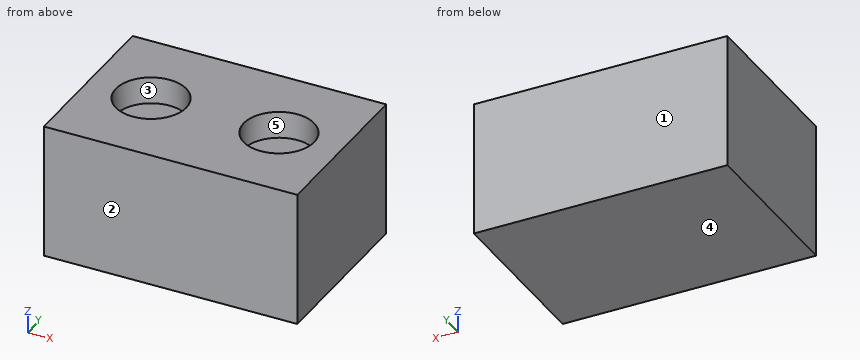
```python
from build123d import *

# Parameters (mm, degrees)
CROQUIS1_W              = 18.8
CROQUIS1_H              = 12.8
SALIENTE_EXTRUIR1_DEPTH = 10
CROQUIS2_R              = 2.614642897
CORTAR_EXTRUIR1_DEPTH   = 2


with BuildPart() as part:
    # Croquis1 → Saliente-Extruir1 (new body)
    with BuildSketch(Plane.XY):
        Rectangle(CROQUIS1_W, CROQUIS1_H)
    extrude(amount=SALIENTE_EXTRUIR1_DEPTH)

    # Croquis2 → Cortar-Extruir1 (cut)
    with BuildSketch(Plane.XY.offset(10)):
        with Locations((-4.740668899, 0)):
            Circle(CROQUIS2_R)
    cortar_extruir1 = extrude(amount=-CORTAR_EXTRUIR1_DEPTH, mode=Mode.SUBTRACT)

    # Simetría1: Cortar-Extruir1 across plane
    add(cortar_extruir1.mirror(Plane(origin=(0, 0, 0), x_dir=(0, 0, 1), z_dir=(1, 0, 0))), mode=Mode.SUBTRACT)


solid = part.part
```
Input: part model. Units: mm. Frame: model coordinates. Face numbers are marked on the shaded views. A direction names the side the tool comes from. Round coordinates to 2 decimals unless told otherwise and drop trailing zeros. Order: outer loops, then holes, each group sorted by start corner. A loop starts at its lowest first (then second) coordinate and runs counter-clockwise, first axis right, second up. Notation, with made-up numbers: (82, 35.25) - (111, 35.25) arc R17 cw to (111, 65.25) - close; hole circle Ø4 at (43.25, 7). An arc over 180 degrees is marked (long way). One line per question, with ' | ' between items. Start each with the question number.
1) Pull-direction query (Y, two-part tool) for the marked faces 1, 2 and 3; classes: +Y half, -Y half, draft (parallel to the pull), parting line (faces both ways), or undercut.
2) Set-up query: the marked faces 4 and 5. Return all of +Z, -Z, +X, -X, +Y, -Y with unobstructed straight access to the full face (end or side cutting, diameter ignored); none if empty.
3) Ray query, probe 1 along Z at (x, y) = (4.25, -0.25); probe 2 along Y at (x, z) = (-6, 9.25). Return the intervals inside material, ascending.
4) Cut plane A-A, the plane z = 9. Return the cut outline in (x, y), then the cut area to 3 significant figures.
5) Contact query for a flat-ended pin moving along its axis: P1, Ø4.5, axis at x = 4.74, y = 0, coming from the +Z side. Output: stop coordinate, or through.
6) Cut plane C-C, the plane x = -2.75. Return the cut outline in (y, z).
7) Cut plane B-B, the plane y = 0. Return the cut outline in (x, z).
Worked out:
1) face 1: +Y half | face 2: -Y half | face 3: undercut
2) face 4: -Z, +X, -X, +Y, -Y | face 5: +Z
3) probe 1: z = 0 to 8 | probe 2: y = -6.4 to -2.29, 2.29 to 6.4
4) outline: (-9.4, -6.4) - (9.4, -6.4) - (9.4, 6.4) - (-9.4, 6.4) - close; hole circle Ø5.23 at (-4.74, 0); hole circle Ø5.23 at (4.74, 0) | area: 198 mm^2
5) P1: stops at z = 8
6) outline: (-6.4, 0) - (6.4, 0) - (6.4, 10) - (1.7, 10) - (1.7, 8) - (-1.7, 8) - (-1.7, 10) - (-6.4, 10) - close
7) outline: (-9.4, 0) - (9.4, 0) - (9.4, 10) - (7.36, 10) - (7.36, 8) - (2.13, 8) - (2.13, 10) - (-2.13, 10) - (-2.13, 8) - (-7.36, 8) - (-7.36, 10) - (-9.4, 10) - close
